Drawing for the job (mm, zero at the part's lowest x, y, z). A direction names the side the tool comes from. Coordinates: 2 decimals unless noted, no trailing zeros. Order: outer loops, then holes, each group sorted by start corner. A loop starts at its lowest first (then second) coordinate and runs counter-clockwise, first axis right, second up.
1) Pin check, flat tips, straight feed: pin 1 Ø1.5 at (y, z) = (11, 27) entering from -X; pin 2 Ø0.9 at (x, y) = (5, 17.5) entering from -Z. Stop position of each tip, or through.
2) Cut at D-D (z = 30.5). List the corners of the cut face in (x, y), and give its area (3 significant figures).
3) Cut at C-C (z = 9). List the corners of the cut face in (x, y).
4) Cut at A-A (y = 17.5). List the corners of the cut face in (x, z), and give its area (3 significant figures).
5) Wall check: L1, parallel to X at y = 17.5, z = 11; L2, parallel to X at y = 5, z = 9.25. Give the ranges that are in metal, low to high.
6) Tool access for the marked faces 1, 2 and 3: list every direction of +Z, -Z, +X, -X, +Y, -Y with a clear straight run to the whole face (end or side of a thin tool).
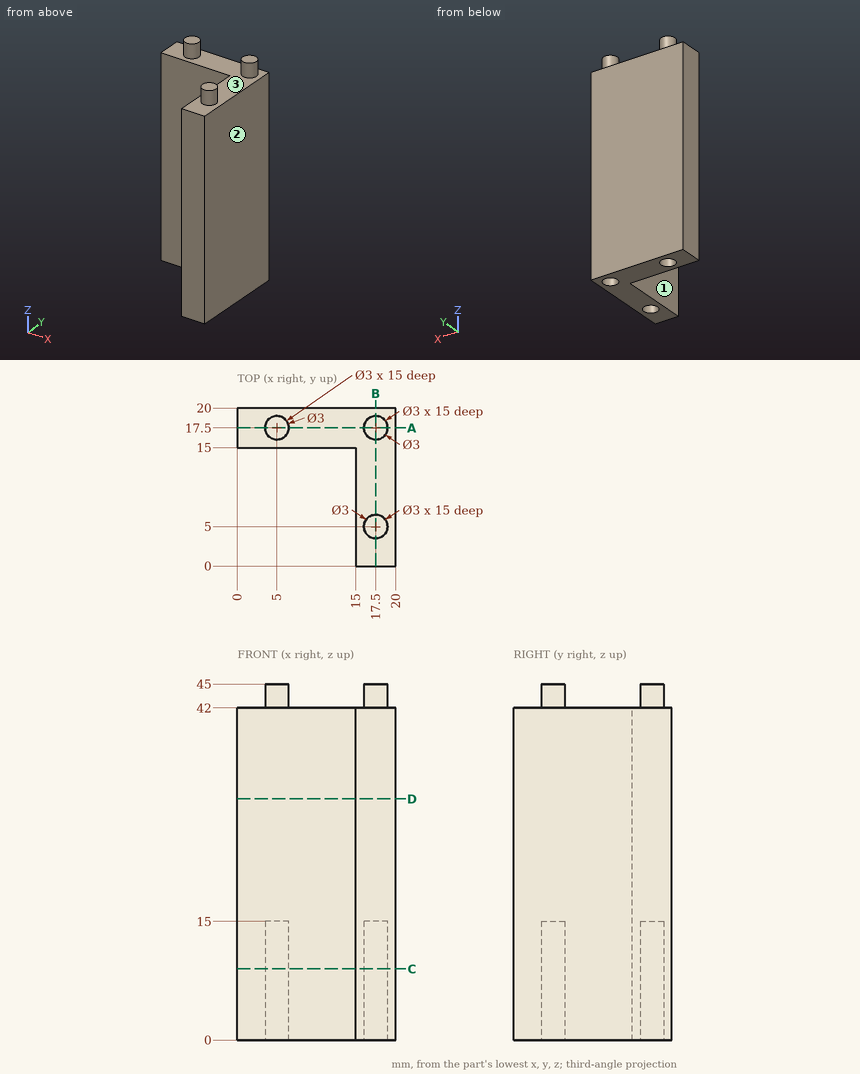
Geometry check:
1. pin 1: stops at x = 15
1. pin 2: stops at z = 15
2. outline: (0, 15) - (15, 15) - (15, 0) - (20, 0) - (20, 20) - (0, 20) - close
2. area: 175 mm2
3. outline: (0, 15) - (15, 15) - (15, 0) - (20, 0) - (20, 20) - (0, 20) - close; hole circle Ø3 at (5, 17.5); hole circle Ø3 at (17.5, 5); hole circle Ø3 at (17.5, 17.5)
4. outline: (0, 0) - (3.5, 0) - (3.5, 15) - (6.5, 15) - (6.5, 0) - (16, 0) - (16, 15) - (19, 15) - (19, 0) - (20, 0) - (20, 42) - (19, 42) - (19, 45) - (16, 45) - (16, 42) - (6.5, 42) - (6.5, 45) - (3.5, 45) - (3.5, 42) - (0, 42) - close
4. area: 768 mm2
5. L1: x = 0 to 3.5, 6.5 to 16, 19 to 20
5. L2: x = 15 to 16, 19 to 20
6. face 1: +Z, -Z, -X, -Y
6. face 2: +Z, -Z, +X, +Y, -Y
6. face 3: +Z
